The model under review builds one solid part; all positions refer to its coordinate system, in mm. Face numbers are marked on the shaded views. A direction names the side the tool comes from. Round coordinates to 2 decimals unless told otherwise and drop trailing zeros. Write each loop counter-clockwise with the first axis right and the second up, starting at its lowest first coordinate (ties: lowest second). Pieces come first, ordered by that corner, then holes. Notation, with made-up numbers: (47, -38.5) -> (69, -38.5) arc R21 ccw to (69, -5.5) -> close; hole circle Ø6 at (-12, 55). An arc over 180 degrees is marked (long way). Return JSON: item names as keys, results as strings. Group by question number.
1. Take a section at D-D, the plane y = 4.5. Write out the cut boundary in (x, z), then the cut area to 3 significant figures.
2. Take a section at B-B, the plane y = 0. Write out the cut boundary in (x, z), then the cut area to 3 significant figures.
3. Clearance check with flat-ended pins moving along their axes: P1, Ø2, axis at y = -1.5, z = 9, coming from the +X side; P2, Ø4, axis at x = -20.47, y = 0, coming from the +Z side; P3, Ø3, axis at y = 2.5, z = 11, coming from the -X side. State where each tip first meets the part, or that it passes through.
4. Take a section at C-C, the plane x = -8. Write out the cut boundary in (y, z).
5. Tool access review of the marked faces 1, 2 and 3: name each direction out of +Z, -Z, +X, -X, +Y, -Y from which nothing blocks a thin tool from reaching the whole face with its end or side.
6. Mouldability with a two-part tool opening along Z and no side actions: class the marked faces 4, 5 and 6 as pulls with the +Z half, pulls with the -Z half, needs draft (parallel to the pull), parting line crosses it, or undercut.
7. For line 1 along Y through (x, z) = (-6, 2.75); line 2 along Z through (x, y) = (22.5, 0.25); line 3 along X through (y, z) = (-3.5, 10.5), list the stretches that pass through material, from the lowest coordinate up. Write a range as from..to.
8. Take a section at A-A, the plane z = 1. Give the number of separate pieces and of enclosed holes in the cut face, then the cut area to 3 significant figures.
from build123d import *

# Parameters (mm, degrees)
SKETCH_W        = 32
SKETCH_H        = 10
PAD_DEPTH       = 14
SKETCH001_R     = 1.5
PAD001_DEPTH    = 3
SKETCH002_W     = 27
SKETCH002_H     = 2
POCKET_DEPTH    = 8
SKETCH003_R     = 0.35
SKETCH003_R_2   = 0.383924
POCKET001_DEPTH = 18
SKETCH004_W     = 1.5
SKETCH004_H     = 6.7
SKETCH004_H_2   = 6.8
SKETCH004_H_3   = 6.771652
POCKET002_DEPTH = 8
SKETCH005_W     = 2
SKETCH005_H     = 1.5
POCKET003_DEPTH = 8
FILLET_R        = 1


with BuildPart() as part:
    # Sketch → Pad (new body)
    with BuildSketch(Plane.XY):
        Rectangle(SKETCH_W, SKETCH_H)
    extrude(amount=PAD_DEPTH)

    # Sketch001 → Pad001 (new body)
    with BuildSketch(Plane(origin=(0, 0, 0), x_dir=(1, 0, 0), z_dir=(0, 0, -1))):
        with BuildLine():
            ThreePointArc((-20.474548, 5), (-25.474548, 0), (-20.474548, -5))
            Line((-20.474548, -5), (20.474548, -5))
            ThreePointArc((20.474548, -5), (25.474548, 0), (20.474548, 5))
            Line((-20.474548, 5), (20.474548, 5))
        make_face()
        with Locations((-20.474548, 0)):
            Circle(SKETCH001_R, mode=Mode.SUBTRACT)
        with Locations((20.474548, 0)):
            Circle(SKETCH001_R, mode=Mode.SUBTRACT)
    extrude(amount=-PAD001_DEPTH)

    # Sketch002 → Pocket (cut)
    with BuildSketch(Plane.XY.offset(14)):
        Rectangle(SKETCH002_W, SKETCH002_H)
    extrude(amount=-POCKET_DEPTH, mode=Mode.SUBTRACT)

    # Sketch003 → Pocket001 (cut)
    with BuildSketch(Plane(origin=(0, 0, 0), x_dir=(1, 0, 0), z_dir=(0, 0, -1))):
        with Locations((-10, 2.25)):
            Circle(SKETCH003_R)
        with Locations((-6, 2.25)):
            Circle(SKETCH003_R)
        with Locations((-2, 2.25)):
            Circle(SKETCH003_R)
        with Locations((2, 2.25)):
            Circle(SKETCH003_R)
        with Locations((6, 2.25)):
            Circle(SKETCH003_R)
        with Locations((10, 2.25)):
            Circle(SKETCH003_R)
        with Locations((-10, -2.25)):
            Circle(SKETCH003_R)
        with Locations((-6, -2.25)):
            Circle(SKETCH003_R)
        with Locations((-2, -2.25)):
            Circle(SKETCH003_R_2)
        with Locations((2, -2.25)):
            Circle(SKETCH003_R)
        with Locations((6, -2.25)):
            Circle(SKETCH003_R)
        with Locations((10, -2.25)):
            Circle(SKETCH003_R)
    extrude(amount=-POCKET001_DEPTH, mode=Mode.SUBTRACT)

    # Sketch004 → Pocket002 (cut)
    with BuildSketch(Plane.XY.offset(14)):
        with Locations((-10, 0)):
            Rectangle(SKETCH004_W, SKETCH004_H)
        with Locations((-6, 0)):
            Rectangle(SKETCH004_W, SKETCH004_H_2)
        with Locations((-2, 0)):
            Rectangle(SKETCH004_W, SKETCH004_H_2)
        with Locations((2, 0)):
            Rectangle(SKETCH004_W, SKETCH004_H_2)
        with Locations((6, 0)):
            Rectangle(SKETCH004_W, SKETCH004_H_2)
        with Locations((10, 0)):
            Rectangle(SKETCH004_W, SKETCH004_H_3)
    extrude(amount=-POCKET002_DEPTH, mode=Mode.SUBTRACT)

    # Sketch005 → Pocket003 (cut)
    with BuildSketch(Plane.XY.offset(14)):
        with Locations((-10, 2.6)):
            Rectangle(SKETCH005_W, SKETCH005_H)
        with Locations((-6, 2.65)):
            Rectangle(SKETCH005_W, SKETCH005_H)
        with Locations((-2, 2.65)):
            Rectangle(SKETCH005_W, SKETCH005_H)
        with Locations((2, 2.65)):
            Rectangle(SKETCH005_W, SKETCH005_H)
        with Locations((6, 2.65)):
            Rectangle(SKETCH005_W, SKETCH005_H)
        with Locations((10, 2.635826)):
            Rectangle(SKETCH005_W, SKETCH005_H)
        with Locations((-10, -2.6)):
            Rectangle(SKETCH005_W, SKETCH005_H)
        with Locations((-6, -2.65)):
            Rectangle(SKETCH005_W, SKETCH005_H)
        with Locations((-2, -2.65)):
            Rectangle(SKETCH005_W, SKETCH005_H)
        with Locations((2, -2.65)):
            Rectangle(SKETCH005_W, SKETCH005_H)
        with Locations((6, -2.65)):
            Rectangle(SKETCH005_W, SKETCH005_H)
        with Locations((10.005354, -2.635826)):
            Rectangle(SKETCH005_W, SKETCH005_H)
    extrude(amount=-POCKET003_DEPTH, mode=Mode.SUBTRACT)

    # Fillet
    fillet_edges = [part.edges().sort_by_distance(p)[0] for p in [
        (-12.125, 1, 14),
        (-8, 1, 14),
        (-4, 1, 14),
        (0, 1, 14),
        (4, 1, 14),
        (8, 1, 14),
        (12.125, 1, 14),
        (12.125, -1, 14),
        (8, -1, 14),
        (4, -1, 14),
        (0, -1, 14),
        (-4, -1, 14),
        (-8, -1, 14),
        (-12.125, -1, 14),
    ]]
    fillet(fillet_edges, radius=FILLET_R)


solid = part.part
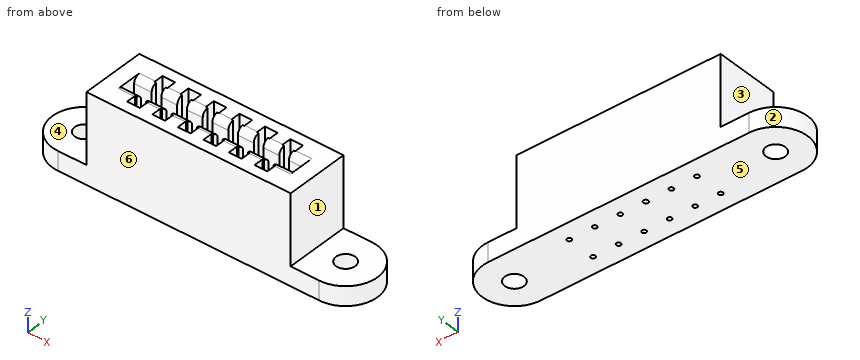
Output:
{
 "1": {"outline": "(-22.65, 0) -> (22.65, 0) -> (22.65, 3) -> (16, 3) -> (16, 14) -> (-16, 14) -> (-16, 3) -> (-22.65, 3) -> close", "area": "488 mm^2"},
 "2": {"outline": "(-25.47, 0) -> (-21.97, 0) -> (-21.97, 3) -> (-25.47, 3) -> close; (-18.97, 0) -> (18.97, 0) -> (18.97, 3) -> (16, 3) -> (16, 14) -> (13.5, 14) -> (13.5, 6) -> (-13.5, 6) -> (-13.5, 14) -> (-16, 14) -> (-16, 3) -> (-18.97, 3) -> close; (21.97, 0) -> (25.47, 0) -> (25.47, 3) -> (21.97, 3) -> close", "area": "271 mm^2"},
 "3": {"P1": "stops at x = 16", "P2": "stops at z = 3", "P3": "stops at x = -16"},
 "4": {"outline": "(-5, 0) -> (5, 0) -> (5, 14) -> (2, 14) arc R1 ccw to (1, 13) -> (1, 6) -> (-1, 6) -> (-1, 13) arc R1 ccw to (-2, 14) -> (-5, 14) -> close"},
 "5": {"face 1": "+Z, +X, +Y, -Y", "face 2": "+Z, -Z, -X", "face 3": "+Z, -X, +Y, -Y"},
 "6": {"face 4": "pulls with the +Z half", "face 5": "pulls with the -Z half", "face 6": "needs draft"},
 "7": {"line 1": "y = -5..-2.6, -1.9..1.9, 2.6..5", "line 2": "z = 0..3", "line 3": "x = -16..16"},
 "8": {"separate pieces": "1", "enclosed holes": "14", "area": "469 mm^2"}
}
